Work out the finished part from the listing and answer in its coordinate system (mm). Coordinates: 2 decimals unless noted, no trailing zeros. Write each loop counter-clockwise with the first axis right and the second up, starting at its lowest first coordinate (ties: lowest second). Pieces come first, ordered by that corner, then holes. Notation, with made-up numbers: (-19.5, 46.25) - (-7.5, 46.25) arc R16 ccw to (-7.5, 52.25) - close; hole circle Ø6 at (55.25, 43.5). An arc over 180 degrees is marked (long way). Use a Markdown table: item, result. Add a question column.
(1) Find the intervals of material crossed by line 1 (Y direction, x = 0, z = 3); line 2 (Y direction, x = 1, z = 2.35); line 3 (X direction, y = -1.5, z = 1.9), in increasing order. Write a range as from..to.
(2) The part is cut by section C-C, the plane y = -13. Give the vertices of the cut face in (x, z).
(3) Given pin 1 Ø1 at (x, z) = (13, 1.5) entering from +Y, flat-ended and moving along its own axis, determine where the tip first touches the part or whether it passes through.
(4) The part is cut by section D-D, the plane z = 3.1. Give the vertices of the cut face in (x, y), then the cut area to 3 significant figures.
(5) The part is cut by section A-A, the plane y = 0. Give the vertices of the cut face in (x, z).
(6) For a pull along Y with two mould halves and no side action, classify faces 1 (the face through (-0.33, 8.84, 2.22)), 2 (the face through (-4, 0, 0)), 3 (the face through (15.24, 6.32, 2.22)) as released by +Y, released by -Y, zero draft, split by the parting line, or undercut.
Autodesk Inventor part; units mm, degrees
ref_plane "YZ Plane" through (0, 0, 0) normal (1, 0, 0) x (0, 1, 0)
ref_plane "XZ Plane" through (0, 0, 0) normal (0, 1, 0) x (-1, 0, 0)
ref_plane "XY Plane" through (0, 0, 0) normal (0, 0, 1) x (1, 0, 0)
sketch "Эскиз1" plane through (0, 0, 0) normal (0, 0, 1) x (1, 0, 0)
  circle A0 centre (0, 0) radius 16.5
  circle A1 centre (0, 0) radius 3.75
  circle A2 centre (0, 0) radius 11.32
  circle A3 centre (-11.32, 0) radius 2.5
  circle A4 centre (0, -11.32) radius 2.5
  circle A5 centre (11.32, 0) radius 2.5
  circle A6 centre (0, 11.32) radius 2.5
  dimension "d2" = 22.64
  dimension "d0" = 33
  dimension "d1" = 7.5
  dimension "d3" = 5
  dimension "d6" = 360
extrude "Выдавливание1" add sketch "Эскиз1" along normal blind 4.5 contours A0 | A5 A2 A4 A3 A6
properties part number "проставка для колеса"
Model answer:
| question | item | result |
|---|---|---|
| 1 | line 1 | -16.5..-13.82, -8.82..-3.75, 3.75..8.82, 13.82..16.5 |
| 1 | line 2 | -16.47..-13.61, -9.03..-3.61, 3.61..9.03, 13.61..16.47 |
| 1 | line 3 | -16.43..-13.32, -9.32..-3.44, 3.44..9.32, 13.32..16.43 |
| 2 | outline | (-10.16, 0) - (-1.85, 0) - (-1.85, 4.5) - (-10.16, 4.5) - close; (1.85, 0) - (10.16, 0) - (10.16, 4.5) - (1.85, 4.5) - close |
| 3 | pin 1 | y = 10.77 |
| 4 | outline | circle Ø33 at (0, 0); hole circle Ø5 at (-11.32, 0); hole circle Ø7.5 at (0, 0); hole circle Ø5 at (0, -11.32); hole circle Ø5 at (0, 11.32); hole circle Ø5 at (11.32, 0) |
| 4 | area | 733 mm^2 |
| 5 | outline | (-16.5, 0) - (-13.82, 0) - (-13.82, 4.5) - (-16.5, 4.5) - close; (-8.82, 0) - (-3.75, 0) - (-3.75, 4.5) - (-8.82, 4.5) - close; (3.75, 0) - (8.82, 0) - (8.82, 4.5) - (3.75, 4.5) - close; (13.82, 0) - (16.5, 0) - (16.5, 4.5) - (13.82, 4.5) - close |
| 6 | face 1 | undercut |
| 6 | face 2 | zero draft |
| 6 | face 3 | split by the parting line |
